from build123d import *

# Parameters (mm, degrees)
BOSS_EXTRUDE1_DEPTH = 30.364999976
BOSS_EXTRUDE2_DEPTH = 21.63499991
SKETCH4_W           = 37.064796383
SKETCH4_H           = 32.7
SKETCH4_R           = 3.625
SKETCH4_R_2         = 1.8
BOSS_EXTRUDE3_DEPTH = 2.5
SKETCH5_R           = 2
CUT_EXTRUDE1_DEPTH  = 7
SKETCH6_R           = 2.000000064
CUT_EXTRUDE2_DEPTH  = 7
CUT_EXTRUDE3_START  = -7
SKETCH7_R           = 2
CUT_EXTRUDE3_DEPTH  = 7


with BuildPart() as part:
    # Sketch1 → Boss-Extrude1 (new body)
    with BuildSketch(Plane.XY):
        with BuildLine():
            Line((23.763847258, 19.05), (23.763847258, 5.4))
            Line((23.763847258, 5.4), (-13.300949125, 5.4))
            Line((-13.300949125, 5.4), (-13.300949125, 19.05))
            Line((-13.300949125, 19.05), (-6.958949124, 19.05))
            ThreePointArc((-6.958949124, 19.05), (5.231449067, 6.859601809), (17.421847257, 19.05))
            Line((17.421847257, 19.05), (23.763847258, 19.05))
        make_face()
    extrude(amount=BOSS_EXTRUDE1_DEPTH)

    # Sketch3 → Boss-Extrude2 (add)
    with BuildSketch(Plane.XY.offset(30.364999976)):
        with BuildLine():
            Line((-13.300949125, 19.05), (-13.300949125, 5.4))
            Line((-13.300949125, 5.4), (23.763847258, 5.4))
            Line((23.763847258, 5.4), (23.763847258, 19.05))
            Line((23.763847258, 19.05), (17.72184715, 19.05))
            ThreePointArc((17.72184715, 19.05), (5.231449012, 6.559601862), (-7.258949126, 19.05))
            Line((-7.258949126, 19.05), (-13.300949125, 19.05))
        make_face()
    extrude(amount=BOSS_EXTRUDE2_DEPTH)

    # Sketch4 → Boss-Extrude3 (add)
    with BuildSketch(Plane.XY.offset(51.999999886)):
        with Locations((5.231449067, 21.75)):
            Rectangle(SKETCH4_W, SKETCH4_H)
        with Locations((5.231449093, 19.05)):
            Circle(SKETCH4_R, mode=Mode.SUBTRACT)
        with Locations((5.231449093, 10.541)):
            Circle(SKETCH4_R_2, mode=Mode.SUBTRACT)
        with Locations((5.231449093, 27.94)):
            Circle(SKETCH4_R_2, mode=Mode.SUBTRACT)
    extrude(amount=BOSS_EXTRUDE3_DEPTH)

    # Sketch5 → Cut-Extrude1 (cut)
    with BuildSketch(Plane.XZ.offset(-5.4)):
        with Locations(Location((-8.220949125, 48.149999886, 0), (0, 0, 270))):
            Circle(SKETCH5_R)
        with Locations(Location((18.683847258, 48.149999886, 0), (0, 0, 270))):
            Circle(SKETCH5_R)
        with Locations(Location((-8.220949125, 6.35, 0), (0, 0, 270))):
            Circle(SKETCH5_R)
        with Locations(Location((18.683847258, 6.35, 0), (0, 0, 270))):
            Circle(SKETCH5_R)
    extrude(amount=-CUT_EXTRUDE1_DEPTH, mode=Mode.SUBTRACT)

    # Sketch6 → Cut-Extrude2 (cut)
    with BuildSketch(Plane.ZY.offset(13.300949125)):
        with Locations(Location((19.05, 11.75, 0), (0, 0, 270))):
            Circle(SKETCH6_R)
    extrude(amount=-CUT_EXTRUDE2_DEPTH, mode=Mode.SUBTRACT)

    # Sketch7 → Cut-Extrude3 (cut)
    with BuildSketch(Plane(origin=(23.763847258, 0, 0), x_dir=(0, 0, -1), z_dir=(1, 0, 0)).offset(CUT_EXTRUDE3_START)):
        with Locations(Location((-19.05, 11.75, 0), (0, 0, 270))):
            Circle(SKETCH7_R)
    extrude(amount=CUT_EXTRUDE3_DEPTH, mode=Mode.SUBTRACT)


solid = part.part
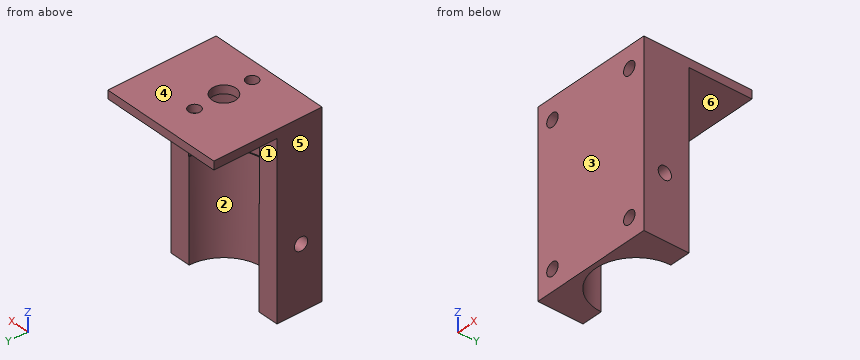
The model under review builds one solid part; all positions refer to its coordinate system, in mm. Face numbers are marked on the shaded views. A direction names the side the tool comes from. Coordinates: 2 decimals unless noted, no trailing zeros. Write each loop counter-clockwise with the first axis right and the second up, starting at its lowest first coordinate (ties: lowest second). Pieces come first, ordered by that corner, then holes. Notation, with made-up numbers: M 77.25,12 L 100.25,12 A19 ccw 100.25,24 Z; hole C 36.5,-5.75 d8. An arc over 180 degrees is marked long. Put each result on its own line as item: value.
1) Add section C-C on z = 6.35. Give the boundary of the cut face in (x, y), then the cut area to 3 significant figures.
Computed:
outline: M -13.3,5.4 L -10.22,5.4 L -10.22,12.4 L -6.22,12.4 L -6.22,5.4 L 16.68,5.4 L 16.68,12.4 L 20.68,12.4 L 20.68,5.4 L 23.76,5.4 L 23.76,19.05 L 17.42,19.05 A12.19 cw -6.96,19.05 L -13.3,19.05 Z
area: 217 mm2
2) Wall thickness on probe 1 along Z at (x, y) = (-9, 9); probe 2 along Y at (x, z) = (20.5, 19.05); probe 3 along Z at (x, y) = (20.5, 23): over which ranges is each line inside the solid? List them lowest first. Write a range as [from, to].
Computed:
probe 1: z = [0, 4.51], [8.19, 46.31], [49.99, 54.5]
probe 2: y = [5.4, 9.75], [13.75, 19.05]
probe 3: z = [52, 54.5]
3) Clearance check with flat-ended pins moving along their axes: pin 1 Ø7 at (x, z) = (-9, 28.5) entering from +Y; pin 2 Ø2 at (y, z) = (20.5, 43) entering from +X; pin 3 Ø6.5 at (x, z) = (-8.22, 48.15) entering from -Y; pin 4 Ø9.5 at (x, y) = (5.23, 19.05) entering from -Z. State where each tip first meets the part, or that it passes through.
Computed:
pin 1: stops at y = 19.05
pin 2: passes through
pin 3: stops at y = 5.4
pin 4: stops at z = 52
4) Add section A-A on y = 11.5. Give the boundary of the cut face in (x, z) (3 decimals).
Computed:
outline: M -13.301,0 L -4.34,0 L -4.34,30.365 L -4.719,30.365 L -4.719,52 L 3.708,52 L 3.708,54.5 L -13.301,54.5 L -13.301,21.034 L -6.301,21.034 L -6.301,17.066 L -13.301,17.066 Z; M 6.755,52 L 15.182,52 L 15.182,30.365 L 14.802,30.365 L 14.802,0 L 23.764,0 L 23.764,17.066 L 16.764,17.066 L 16.764,21.034 L 23.764,21.034 L 23.764,54.5 L 6.755,54.5 Z; hole C -8.221,6.35 d4; hole C -8.221,48.15 d4; hole C 18.684,6.35 d4; hole C 18.684,48.15 d4
5) Add section D-D on x = 14. Give the boundary of the cut face in (y, z) (3 decimals), then the cut area to 3 significant figures.
Computed:
outline: M 5.4,0 L 10.581,0 L 10.581,30.365 L 10.155,30.365 L 10.155,52 L 38.1,52 L 38.1,54.5 L 5.4,54.5 Z
area: 342 mm2
6) Draft analysis for pull direction X (two halves, no side actions). For the marked faces 4, 5 and 6, state which applies: released by +X, released by -X, zero draft, split by the parting line, or undercut.
Computed:
face 4: zero draft
face 5: released by -X
face 6: undercut
7) For the marked faces 1, 2 and 3, list the 3-axis set-ups (+Z, -Z, +X, -X, +Y, -Y) from which the entire face can be reached by the end or side of a thin tool; tool diameter is ignored.
Computed:
face 1: -Z, +X, -X, +Y
face 2: -Z, +Y
face 3: +Z, -Z, +X, -X, -Y
8) Add section B-B on y = 27.94. Give the boundary of the cut face in (x, z).
Computed:
outline: M -13.3,52 L 3.43,52 L 3.43,54.5 L -13.3,54.5 Z; M 7.03,52 L 23.76,52 L 23.76,54.5 L 7.03,54.5 Z
